Geometry check sheet. Reference: drawing and pictorial views, mm from the part's lowest x, y, z. A direction names the side the tool comes from. Give positions to 0.01 mm unless a question says otherwise; leave off trailing zeros. Write each loop counter-clockwise with the first axis right and the second up, starting at its lowest first coordinate (ties: lowest second). Pieces come first, ordered by that corner, then holes. Notation, with made-up numbers: (17.25, 55.25) - (50.25, 55.25) arc R17 ccw to (50.25, 72.25) - close; hole circle Ø10 at (-18, 46). An arc over 180 degrees is marked (long way). Put each result on its own line as item: value.
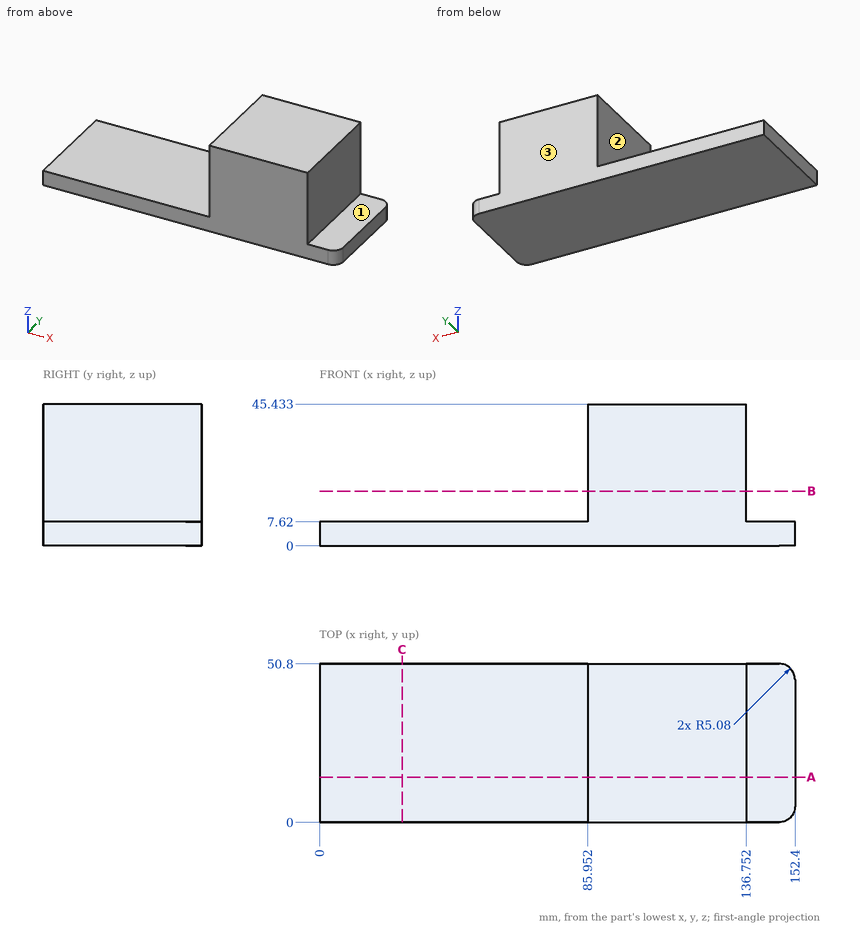
Q1. Set-up check for the marked faces 1, 2 and 3: record each of +Z, -Z, +X, -X, +Y, -Y from which the full face is reachable in a straight line by a thin tool's end or side.
Answers follow:
face 1: +Z, +X, +Y, -Y
face 2: +Z, -X, +Y, -Y
face 3: +Z, -Z, +X, -X, +Y
Q2. Go/stop test with flat-tipped pins: pin 1 Ø15 at (x, y) = (34, 31.5) entering from +Z; pin 2 Ø4 at (y, z) = (42, 17) entering from +X; pin 3 Ø1 at (y, z) = (32, 37.5) entering from -X. Record where each tip stops, or that it passes through.
Answers follow:
pin 1: stops at z = 7.62
pin 2: stops at x = 136.75
pin 3: stops at x = 85.95
Q3. Section check C-C, the plane x = 26.5. Record the cut outline in (y, z), plus the area to 3 significant figures.
Answers follow:
outline: (0, 0) - (50.8, 0) - (50.8, 7.62) - (0, 7.62) - close
area: 387 mm2
Q4. Section check B-B, the plane z = 17.5. Record the cut outline in (x, y).
Answers follow:
outline: (85.95, 0) - (136.75, 0) - (136.75, 50.8) - (85.95, 50.8) - close
Q5. Scan lines: line 1 along Z through (x, y) = (34, 43); line 2 along X through (y, z) = (26, 26.5). Record each from-to range of solid material in increasing order.
Answers follow:
line 1: z = 0 to 7.62
line 2: x = 85.95 to 136.75
Q6. Section check A-A, the plane y = 14.5. Record the cut outline in (x, z).
Answers follow:
outline: (0, 0) - (152.4, 0) - (152.4, 7.62) - (136.75, 7.62) - (136.75, 45.43) - (85.95, 45.43) - (85.95, 7.62) - (0, 7.62) - close
